Geometry check sheet. Reference: the model listing, model coordinates, mm. Coordinates: 2 decimals unless noted, no trailing zeros. Write each loop counter-clockwise with the first axis right and the second up, starting at its lowest first coordinate (ties: lowest second). Pieces come first, ordered by that corner, then holes. Notation, with made-up numbers: M 51,76 L 63,76 A36 ccw 63,111 Z; hole C 38.25,23 d2. An arc over 180 degrees is marked long. Answer as a JSON object with one key per item and string values. Group by question number.
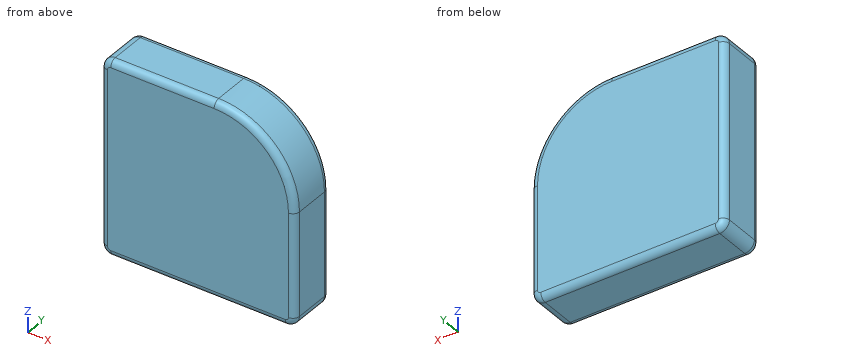
```python
from build123d import *

# Parameters (mm, degrees)
F1_DEPTH = 15
F2_R     = 2
F3_R     = 2


with BuildPart() as f1:
    # F0 (on Front) → F1 (new body)
    with BuildSketch(Plane.XZ):
        with BuildLine():
            Line((-57, 0), (-3, 0))
            ThreePointArc((-3, 0), (-0.87868, 0.87868), (0, 3))
            Line((0, 3), (0, 35))
            ThreePointArc((0, 35), (-7.32233, 52.67767), (-25, 60))
            Line((-25, 60), (-57, 60))
            ThreePointArc((-57, 60), (-59.12132, 59.12132), (-60, 57))
            Line((-60, 57), (-60, 3))
            ThreePointArc((-60, 3), (-59.12132, 0.87868), (-57, 0))
        make_face()
    extrude(amount=F1_DEPTH)

    # F2
    f2_edges = [f1.edges().sort_by_distance(p)[0] for p in [
        (-30, -15, 0),
        (-0.87868, -15, 0.87868),
        (0, -15, 19),
        (-7.32233, -15, 52.67767),
        (-41, -15, 60),
        (-59.12132, -15, 59.12132),
        (-60, -15, 30),
        (-59.12132, -15, 0.87868),
    ]]
    fillet(f2_edges, radius=F2_R)

    # F3
    f3_edges = [f1.edges().sort_by_distance(p)[0] for p in [
        (-41, 0, 60),
    ]]
    fillet(f3_edges, radius=F3_R)


solid = f1.part
```
1) Go/stop test with flat-tipped pins: pin 1 Ø2 at (x, y) = (-12.5, -6.5) entering from +Z; pin 2 Ø2 at (y, z) = (-13, 48) entering from +X. Record where each tip stops, or that it passes through.
2) Material ranges on probe 1 along X at (y, z) = (-2.5, 35.5) (3 decimals); probe 2 along X at (y, z) = (-0.25, 46) (3 decimals); probe 3 along Z at (x, y) = (-15, -6.5), recorded low to high. Write a range as [from, to].
3) Section check A-A (y = -10.25). Record the cut outline in (x, z).
Entries:
{
 "1": {"pin 1": "z = 57.2", "pin 2": "x = -3.07"},
 "2": {"probe 1": "[-60, -0.005]", "probe 2": "[-58.968, -3.705]", "probe 3": "[0, 57.91]"},
 "3": {"outline": "M -60,3 A3 ccw -57,0 L -3,0 A3 ccw 0,3 L 0,35 A25 ccw -25,60 L -57,60 A3 ccw -60,57 Z"}
}
